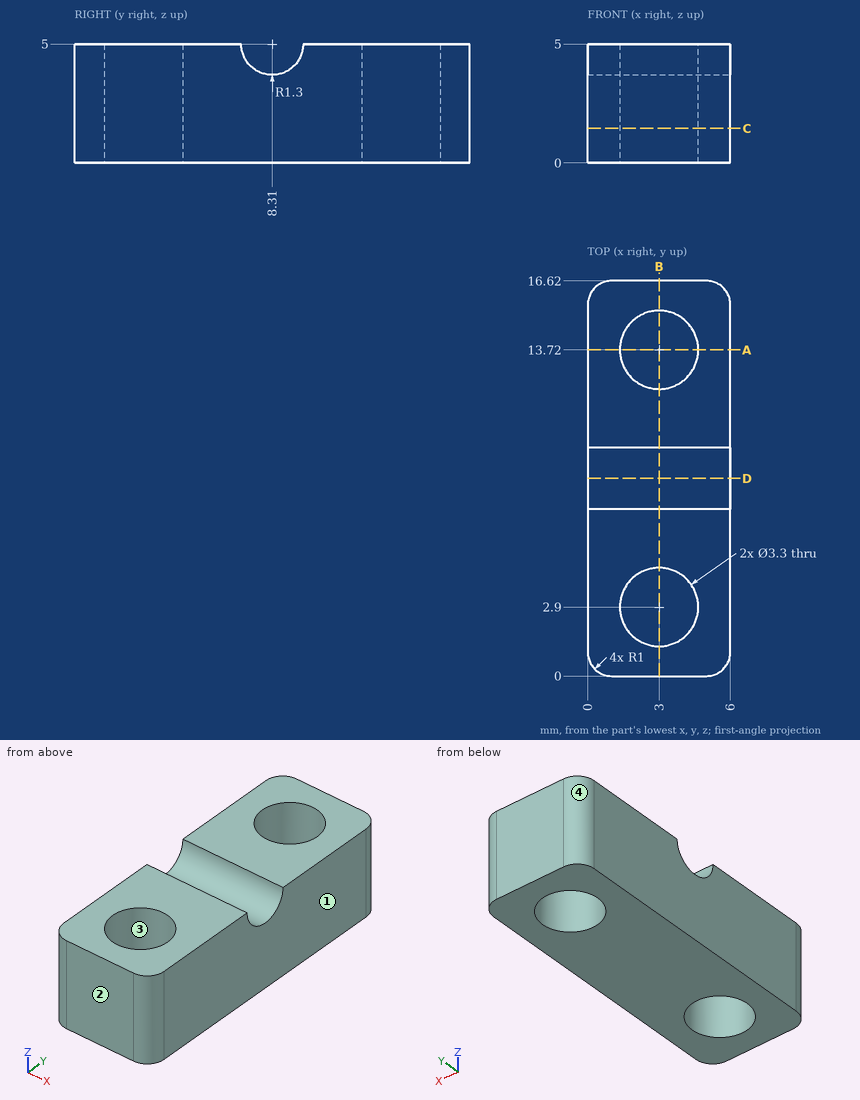
Check sheet for the drawn part. Datum: minimum x, y, z corner. Units: mm. Round coordinates to 2 decimals unless told otherwise and drop trailing zeros. Order: outer loops, then holes, each group sorted by start corner. A loop starts at its lowest first (then second) coordinate and runs counter-clockwise, first axis right, second up.
1. Section check D-D on y = 8.31. Record the cut outline in (x, z), then the cut area to 3 significant figures.
Final values:
outline: (0, 0) - (6, 0) - (6, 3.7) - (0, 3.7) - close
area: 22.2 mm2
2. Section check A-A on y = 13.72. Record the cut outline in (x, z), then the cut area to 3 significant figures.
Final values:
outline: (0, 0) - (1.35, 0) - (1.35, 5) - (0, 5) - close; (4.65, 0) - (6, 0) - (6, 5) - (4.65, 5) - close
area: 13.5 mm2
3. Section check B-B on x = 3. Record the cut outline in (y, z).
Final values:
outline: (0, 0) - (1.25, 0) - (1.25, 5) - (0, 5) - close; (4.55, 0) - (12.07, 0) - (12.07, 5) - (9.61, 5) arc R1.3 cw to (7.01, 5) - (4.55, 5) - close; (15.37, 0) - (16.62, 0) - (16.62, 5) - (15.37, 5) - close
4. Release check for a two-part mould opening along Y. For the marked faces 1, 2, 3 and 4 record: +Y half, -Y half, draft (parallel to the pull), parting line (faces both ways), or undercut.
Final values:
face 1: draft
face 2: -Y half
face 3: undercut
face 4: +Y half
5. Thickness scan on L1, parallel to Y at x = 3, z = 3.65; L2, parallel to Y at x = 2.35, z = 1.6; L3, parallel to X at y = 13.5, z = 4.8. Record the ranges inside material, lowest first.
Final values:
L1: y = 0 to 1.25, 4.55 to 12.07, 15.37 to 16.62
L2: y = 0 to 1.38, 4.42 to 12.2, 15.24 to 16.62
L3: x = 0 to 1.36, 4.64 to 6
6. Section check C-C on z = 1.45. Record the cut outline in (x, y), then the cut area to 3 significant figures.
Final values:
outline: (0, 1) arc R1 ccw to (1, 0) - (5, 0) arc R1 ccw to (6, 1) - (6, 15.62) arc R1 ccw to (5, 16.62) - (1, 16.62) arc R1 ccw to (0, 15.62) - close; hole circle Ø3.3 at (3, 2.9); hole circle Ø3.3 at (3, 13.72)
area: 81.8 mm2
